Input: part model. Units: mm. Frame: model coordinates. Face numbers are marked on the shaded views. A direction names the side the tool comes from. Coordinates: 2 decimals unless noted, no trailing zeros. Order: outer loops, then holes, each group sorted by start corner. A loop starts at its lowest first (then second) coordinate and runs counter-clockwise, first axis right, second up. Notation, with made-up numbers: (-22.75, 27) -> (29.25, 27) arc R28 ccw to (29.25, 65) -> close; hole circle Ø3 at (-31.5, 43.5). An arc over 180 degrees is marked (long way). Answer as CSV lines item,"result".
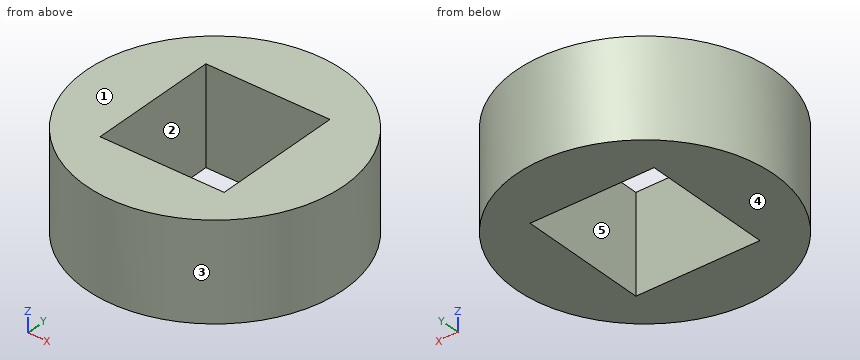
from build123d import *

# Parameters (mm, degrees)
F0_W     = 30.617888
F0_H     = 32.374126
F1_DEPTH = 25
F2_R     = 31.82383
F3_DEPTH = 24


with BuildPart() as f1:
    # F0 (on Top) → F1 (new body)
    with BuildSketch(Plane.XY):
        Rectangle(F0_W, F0_H)
    extrude(amount=F1_DEPTH)


with BuildPart() as f3:
    # F2 (on Top) → F3 (new body)
    with BuildSketch(Plane.XY):
        Circle(F2_R)
    extrude(amount=F3_DEPTH)

    # F4: cut F1
    add(f1.part, mode=Mode.SUBTRACT)


solid = f3.part
1. Contact query for flat-ended pins moving along their axis: pin 1 (12 mm diameter, centred on x = -7, z = 10.5, fed in from +Y); pin 2 (8 mm diameter, centred on x = 21.5, z = 17.5, fed in from +Y); pin 3 (3 mm diameter, centred on x = -22.5, z = 15.5, fed in from +Y). Output: stop coordinate, or through.
Findings:
pin 1,"stops at y = 31.81"
pin 2,"stops at y = 26.58"
pin 3,"stops at y = 23.91"
2. Reachability of the marked faces 1 and 2 from +Z, -Z, +X, -X, +Y, -Y: full face, straight path, thin tool, end or side. Return the list, or none.
Findings:
face 1,"+Z, +X, -X, +Y, -Y"
face 2,"+Z, -Z"
3. Cut plane B-B (x = 0). Return the cut outline in (y, z).
Findings:
outline,"(-31.82, 0) -> (-16.19, 0) -> (-16.19, 24) -> (-31.82, 24) -> close; (16.19, 0) -> (31.82, 0) -> (31.82, 24) -> (16.19, 24) -> close"
4. Ray query, line 1 along Y through (x, z) = (-0.5, 22.25); line 2 along Y through (x, z) = (-13, 9.5); line 3 along X through (y, z) = (-1.5, 6.5). Return the intervals inside material, ascending.
Findings:
line 1,"y = -31.82 to -16.19, 16.19 to 31.82"
line 2,"y = -29.05 to -16.19, 16.19 to 29.05"
line 3,"x = -31.79 to -15.31, 15.31 to 31.79"
5. Mould query, pull axis X, two halves, no side actions, for the marked faces 3, 4 and 5. Classes: released by +X, released by -X, zero draft, split by the parting line, or undercut.
Findings:
face 3,"split by the parting line"
face 4,"zero draft"
face 5,"undercut"
6. Cut plane A-A (y = 0). Return the cut outline in (x, z).
Findings:
outline,"(-31.82, 0) -> (-15.31, 0) -> (-15.31, 24) -> (-31.82, 24) -> close; (15.31, 0) -> (31.82, 0) -> (31.82, 24) -> (15.31, 24) -> close"
7. Cut plane C-C (z = 21.75). Return the cut outline in (x, y).
Findings:
outline,"circle Ø63.65 at (0, 0); hole (-15.31, -16.19) -> (15.31, -16.19) -> (15.31, 16.19) -> (-15.31, 16.19) -> close"
